Part print with two shaded views. Sizes in mm from the minimum x, y, z corner. Give positions to 0.01 mm unless a question says otherwise; leave off trailing zeros. Order: outer loops, then holes, each group sorted by start corner. A loop starts at its lowest first (then second) coordinate and runs counter-clockwise, first axis right, second up. Notation, with made-up numbers: (46, -24.5) -> (85, -24.5) arc R9 ccw to (85, -7.5) -> close; hole circle Ø4 at (45.5, 30.5). An arc over 180 degrees is marked (long way). Answer as CSV lines item,"result".
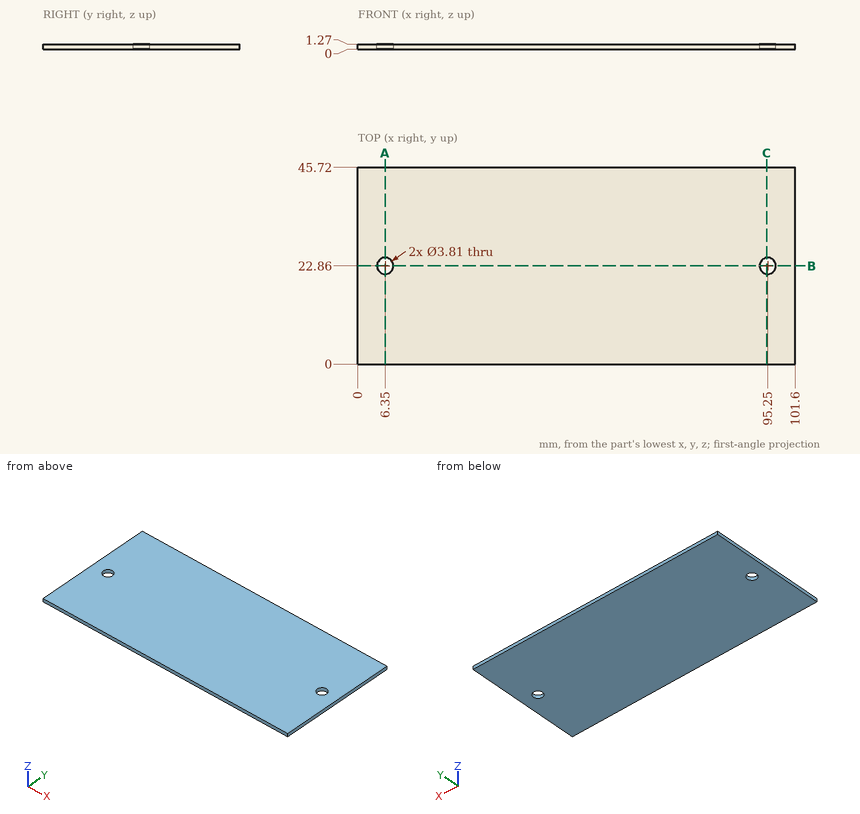
1) Band-saw the part on A-A, the plane x = 6.35. Write the cut outline in (y, z) (3 decimals), then the cut area to 3 significant figures.
Data:
outline,"(0, 0) -> (20.955, 0) -> (20.955, 1.27) -> (0, 1.27) -> close; (24.765, 0) -> (45.72, 0) -> (45.72, 1.27) -> (24.765, 1.27) -> close"
area,"53.2 mm2"
2) Band-saw the part on B-B, the plane y = 22.86. Write the cut outline in (x, z) (3 decimals), then the cut area to 3 significant figures.
Data:
outline,"(0, 0) -> (4.445, 0) -> (4.445, 1.27) -> (0, 1.27) -> close; (8.255, 0) -> (93.345, 0) -> (93.345, 1.27) -> (8.255, 1.27) -> close; (97.155, 0) -> (101.6, 0) -> (101.6, 1.27) -> (97.155, 1.27) -> close"
area,"119 mm2"
3) Wall check: line 1 along X through (y, z) = (23, 0.7); line 2 along Y through (x, z) = (95.25, 0.35) (3 decimals); line 3 along Y through (x, z) = (93.5, 0.55). Give the ranges that are in metal, low to high. Write a range as [from, to].
Data:
line 1,"x = [0, 4.45], [8.25, 93.35], [97.15, 101.6]"
line 2,"y = [0, 20.955], [24.765, 45.72]"
line 3,"y = [0, 22.11], [23.61, 45.72]"
4) Band-saw the part on C-C, the plane x = 95. Write the cut outline in (y, z).
Data:
outline,"(0, 0) -> (20.97, 0) -> (20.97, 1.27) -> (0, 1.27) -> close; (24.75, 0) -> (45.72, 0) -> (45.72, 1.27) -> (24.75, 1.27) -> close"
5) Pin check, flat tips, straight feed: P1, Ø1, axis at x = 36, y = 40, coming from the -Z side; P2, Ø3.5, axis at x = 95.25, y = 22.86, coming from the +Z side. Stop position of each tip, or through.
Data:
P1,"stops at z = 0"
P2,"passes through"
